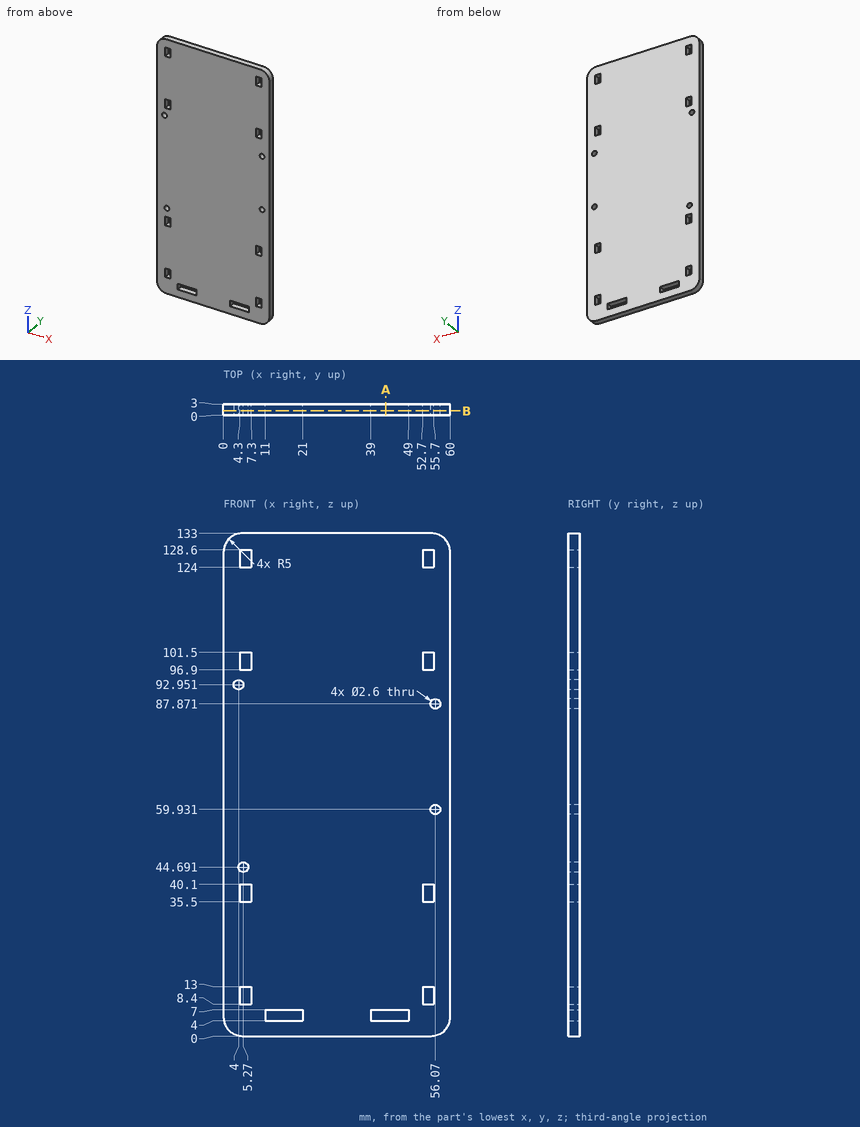
Print and shaded views of the part. All mm, measured from the part's lowest x, y and z. Coordinates: 2 decimals unless noted, no trailing zeros. Loops run counter-clockwise (first coordinate to the right, second up) from the corner with the lowest first, then second, coordinate; pieces in that order, holes last. Notation, with made-up numbers: M 33.25,38.25 L 91.25,38.25 A14 cw 91.25,63.25 Z; hole C 58.5,22.25 d4. An arc over 180 degrees is marked long. Use a Markdown table: item, result. Add a question column.
Q1. Cut at B-B (y = 1.15). Give the number of separate pieces and of enclosed holes in the cut face, and give its area (3 significant figures).
Q2. Probe L1, parallel to X at y = 0.75, z = 6.5; L2, parallel to X at y = 0.6, z = 93; L3, parallel to Z at x = 18, y = 1. List the from-to ranges inside material, lowest first.
Q3. Cut at A-A (x = 43). Write the cut outline in (y, z).
Q4. Pin check, flat tip, straight feed: P1, Ø2, axis at x = 12, z = 91.5, coming from the -Y side. Stop position of the tip, or through.
Worked out:
| question | item | result |
|---|---|---|
| 1 | separate pieces | 1 |
| 1 | enclosed holes | 14 |
| 1 | area | 7,770 mm2 |
| 2 | L1 | x = 0 to 11, 21 to 39, 49 to 60 |
| 2 | L2 | x = 0 to 2.7, 5.3 to 60 |
| 2 | L3 | z = 0 to 4, 7 to 133 |
| 3 | outline | M 0,0 L 3,0 L 3,4 L 0,4 Z; M 0,7 L 3,7 L 3,133 L 0,133 Z |
| 4 | P1 | stops at y = 0 |
